For this review, take the finished solid that the model builds, in its own axes (mm). A direction names the side the tool comes from. Coordinates: 2 decimals unless noted, no trailing zeros. Loops run counter-clockwise (first coordinate to the right, second up) from the corner with the lowest first, then second, coordinate; pieces in that order, holes last. Notation, with made-up numbers: (-16, -37) -> (-11, -37) arc R19 cw to (-11, -17) -> close; hole circle Ø11 at (86, 15.5). An arc over 180 degrees is marked (long way). One line per item, written item: value.
from build123d import *

# Parameters (mm, degrees)
BOSS_EXTRUDE1_DEPTH        = 4.7625
SKETCH3_R                  = 2.05
CUT_EXTRUDE1_DEPTH         = 46.128865832
SKETCH4_R                  = 4.7625
CUT_EXTRUDE2_DEPTH         = 38.1
SKETCH5_W                  = 25.4
SKETCH5_H                  = 25.4
BOSS_EXTRUDE2_DEPTH        = 1.5875
SKETCH6_W                  = 23.891441553
SKETCH6_H                  = 12.7
CUT_EXTRUDE3_DEPTH         = 0.762
FILLET1_R                  = 1.27
F_2_56_TAPPED_HOLE1_REACH  = 32.432
F_2_56_TAPPED_HOLE1_BORE_R = 0.889


with BuildPart() as part:
    # Sketch2 → Boss-Extrude1 (new, symmetric)
    with BuildSketch(Plane(origin=(0, 0, 0), x_dir=(0, 0, -1), z_dir=(1, 0, 0))):
        Polygon((-4.7625, 12.7), (3, 12.7), (3, -25.4), (6.175, -25.4), (6.175, 19.05), (-4.7625, 19.05), align=None)
    extrude(amount=BOSS_EXTRUDE1_DEPTH, both=True)

    # Sketch3 → Cut-Extrude1 (cut, through all)
    with BuildSketch(Plane(origin=(0, 19.05, 0), x_dir=(1, 0, 0), z_dir=(0, 1, 0))):
        with Locations(Location((0, 0, 0), (0, 0, 270))):
            Circle(SKETCH3_R)
    extrude(amount=-CUT_EXTRUDE1_DEPTH, mode=Mode.SUBTRACT)

    # Sketch4 → Cut-Extrude2 (cut)
    with BuildSketch(Plane.XZ.offset(25.4)):
        with Locations((0, 1.0005)):
            Circle(SKETCH4_R)
    extrude(amount=-CUT_EXTRUDE2_DEPTH, mode=Mode.SUBTRACT)

    # Sketch5 → Boss-Extrude2 (add)
    with BuildSketch(Plane(origin=(0, 0, -6.175), x_dir=(-1, 0, 0), z_dir=(0, 0, -1))):
        with Locations((0, -12.7)):
            Rectangle(SKETCH5_W, SKETCH5_H)
    extrude(amount=-BOSS_EXTRUDE2_DEPTH)

    # Sketch6 → Cut-Extrude3 (cut)
    with BuildSketch(Plane.XY.offset(-3)):
        with Locations((3.216659965, 6.35)):
            Rectangle(SKETCH6_W, SKETCH6_H)
    extrude(amount=-CUT_EXTRUDE3_DEPTH, mode=Mode.SUBTRACT)

    # Fillet1
    fillet1_edges = [part.edges().sort_by_distance(p)[0] for p in [
        (4.7625, 15.875, 4.7625),
        (-4.7625, 0, -5.38125),
        (-12.7, -25.4, -5.38125),
        (-12.7, 0, -5.38125),
        (12.7, -25.4, -5.38125),
        (4.7625, 0, -5.38125),
        (0, 12.7, -3.762),
        (-4.7625, 15.875, 4.7625),
    ]]
    fillet(fillet1_edges, radius=FILLET1_R)

    # #2-56 Tapped Hole1 bore → #2-56 Tapped Hole1 (cut, up to next)
    with BuildSketch(Plane.XY.offset(4.7625), mode=Mode.PRIVATE) as f_2_56_tapped_hole1_sk1:
        with Locations((0, 15.875)):
            Circle(F_2_56_TAPPED_HOLE1_BORE_R)
    f_2_56_tapped_hole1_tool1 = extrude(f_2_56_tapped_hole1_sk1.sketch, amount=-F_2_56_TAPPED_HOLE1_REACH, mode=Mode.PRIVATE) & part.part
    add(f_2_56_tapped_hole1_tool1.solids().sort_by_distance((0, 15.875, 4.7625))[0], mode=Mode.SUBTRACT)


solid = part.part
1. Insertion check: pin 1 Ø2 at (x, y) = (-7.5, 14.5) entering from -Z; pin 2 Ø2.5 at (x, y) = (10, -12.5) entering from +Z; pin 3 Ø1.7 at (x, y) = (3, -17) entering from +Z; pin 4 Ø0.5 at (x, z) = (9, -5.5) entering from +Y. Each pin has a flat end and moves straight along its axis. Give the tip position at first contact, or say it passes through.
Return value:
pin 1: passes through
pin 2: stops at z = -4.59
pin 3: stops at z = -3
pin 4: stops at y = 0
2. Take a section at B-B, the plane y = -6. Give the boundary of the cut face in (x, z) (1 decimal), and give its area (3 significant figures).
Return value:
outline: (-12.7, -6.2) -> (12.7, -6.2) -> (12.7, -4.6) -> (4.8, -4.6) -> (4.8, -3) -> (2.6, -3) arc R4.8 cw to (-2.6, -3) -> (-4.8, -3) -> (-4.8, -4.6) -> (-12.7, -4.6) -> close
area: 52.8 mm2
3. To check wall thickness, follow probe 1 along Y at (x, z) = (0, 4.2); probe 2 along X at (y, z) = (15.75, 0); probe 3 along Z at (x, y) = (10.25, -17) (1 decimal). State the ranges of each line that lie inside material, in increasing order. Write a range as from..to.
Return value:
probe 1: y = 12.7..14.99, 16.76..19.05
probe 2: x = -4.76..-2.05, 2.05..4.76
probe 3: z = -6.2..-4.6
4. The part is to be moulded in two halves that separate along Y. For faces 1 (the cylindrical face through (0.09, 15.92, -2.05)), 2 (the cylindrical face through (5.125, 0.382, -5.392)), 3 (the flat face through (1, 12.7, 2)), 4 (the cylindrical face through (0.07, 12.32, -3.4)), say which applies: pulls with the +Y half, pulls with the -Y half, needs draft (parallel to the pull), parting line crosses it, or undercut.
Return value:
face 1: needs draft
face 2: pulls with the +Y half
face 3: pulls with the -Y half
face 4: undercut
5. Take a section at D-D, the plane z = 4. Give the boundary of the cut face in (x, y) (3 decimals).
Return value:
outline: (-4.657, 12.7) -> (4.657, 12.7) -> (4.657, 19.05) -> (-4.657, 19.05) -> close; hole circle Ø1.778 at (0, 15.875)
6. Take a section at C-C, the plane x = 4.25. Give the boundary of the cut face in (y, z) (3 decimals), and give its area (3 significant figures).
Return value:
outline: (-25.4, -6.175) -> (19.05, -6.175) -> (19.05, 4.512) -> (12.7, 4.512) -> (12.7, -2.492) arc R1.27 cw to (11.43, -3.762) -> (0, -3.762) -> (0, -3) -> (-25.4, -3) -> close
area: 179 mm2
7. Take a section at A-A, the plane z = 0. Give the boundary of the cut face in (x, y).
Return value:
outline: (-4.76, 12.7) -> (-2.05, 12.7) -> (-2.05, 19.05) -> (-4.76, 19.05) -> close; (2.05, 12.7) -> (4.76, 12.7) -> (4.76, 19.05) -> (2.05, 19.05) -> close
8. For faces 5 (the flat face through (-9, 0, -5)), 6 (the flat face through (-4.762, 5, -4)), 7 (the flat face through (4.762, 5, -4)), list the 3-axis set-ups (+Z, -Z, +X, -X, +Y, -Y) from which the entire face can be reached by the end or side of a thin tool; tool diameter is ignored.
Return value:
face 5: +Z, -Z, -X, +Y
face 6: +Z, -X, +Y
face 7: +Z, +X, +Y
